```python
from build123d import *

# Parameters (mm, degrees)
LINEAR_AUSTRAGEN1_DEPTH         = 5
M5X0_8_GEWINDEKERNLOCH1_D       = 4.2
M5X0_8_GEWINDEKERNLOCH1_DEPTH   = 14
M5X0_8_GEWINDEKERNLOCH1_TIP     = 1.2618073
SKIZZE5_R                       = 2.5
SCHNITT_LINEAR_AUSTRAGEN1_DEPTH = 825.102693843
LINEARES_MUSTER1_COUNT          = 2
LINEARES_MUSTER1_PITCH          = 60
LINEARES_MUSTER1_COUNT_DIR2     = 2
LINEARES_MUSTER1_PITCH_DIR2     = 75


with BuildPart() as part:
    # Skizze1 → Linear austragen1 (new body)
    with BuildSketch(Plane.XY):
        Polygon((-370.5, 400), (370.5, 400), (370.5, 348), (422.5, 348), (422.5, 360), (708.5, 360), (708.5, 348), (720.5, 348), (720.5, -348), (708.5, -348), (708.5, -360), (422.5, -360), (422.5, -348), (370.5, -348), (370.5, -400), (-370.5, -400), align=None)
    extrude(amount=LINEAR_AUSTRAGEN1_DEPTH)

    # M5x0.8 Gewindekernloch1
    with Locations(Plane(origin=(345.5, 206, 5), x_dir=(1, 0, 0), z_dir=(0, 0, 1))):
        with Locations((0, 0), (-100, 0), (-100, -100), (0, -100), (0, -312), (-100, -312), (0, -412), (-100, -412)):
            Hole(M5X0_8_GEWINDEKERNLOCH1_D / 2, depth=M5X0_8_GEWINDEKERNLOCH1_DEPTH)
            with Locations((0, 0, -(M5X0_8_GEWINDEKERNLOCH1_DEPTH + M5X0_8_GEWINDEKERNLOCH1_TIP / 2))):  # 118° drill point
                Cone(0, M5X0_8_GEWINDEKERNLOCH1_D / 2, M5X0_8_GEWINDEKERNLOCH1_TIP, mode=Mode.SUBTRACT)

    # Skizze5 → Schnitt-Linear austragen1 (cut, through all)
    with BuildSketch(Plane.XY.offset(5)):
        with Locations((240.5, 183)):
            Circle(SKIZZE5_R)
        with Locations((240.5, 129.152)):
            Circle(SKIZZE5_R)
        with Locations((240.5, -128.952)):
            Circle(SKIZZE5_R)
        with Locations((240.5, -182.8)):
            Circle(SKIZZE5_R)
    extrude(amount=-SCHNITT_LINEAR_AUSTRAGEN1_DEPTH, mode=Mode.SUBTRACT)

    # Skizze8 → Ø6.5 (6.5) Durchmesser Bohrung1 (revolve, cut)
    with BuildSketch(Plane(origin=(427.5, 186, 5), x_dir=(0, -1, 0), z_dir=(1, 0, 0))):
        Polygon((0, 0), (0, 21.952797012), (3.25, 20), (3.25, 0), align=None)
    f_6_5_6_5_durchmesser_bohrung1 = revolve(axis=Axis((427.5, 186, 11.35), (0, 0, -1)), mode=Mode.SUBTRACT)

    # Lineares Muster1: 6.5 _6.5_ Durchmesser Bohrung1 2 × 2
    with Locations(*[(j * LINEARES_MUSTER1_PITCH_DIR2, -i * LINEARES_MUSTER1_PITCH, 0) for i in range(LINEARES_MUSTER1_COUNT) for j in range(LINEARES_MUSTER1_COUNT_DIR2) if (i, j) != (0, 0)]):
        add(f_6_5_6_5_durchmesser_bohrung1, mode=Mode.SUBTRACT)

    # Spiegeln1: Ø6.5 (6.5) Durchmesser Bohrung1 across plane
    add(f_6_5_6_5_durchmesser_bohrung1.mirror(Plane.ZX), mode=Mode.SUBTRACT)

    # Spiegeln1 copy 1 sketch → Spiegeln1 copy 1 (revolve, cut)
    with BuildSketch(Plane(origin=(502.5, -186, 5), x_dir=(0, 1, 0), z_dir=(1, 0, 0))):
        Polygon((0, 0), (0, -21.952797012), (3.25, -20), (3.25, 0), align=None)
    revolve(axis=Axis((502.5, -186, 11.35), (0, 0, 1)), mode=Mode.SUBTRACT)

    # Spiegeln1 copy 2 sketch → Spiegeln1 copy 2 (revolve, cut)
    with BuildSketch(Plane(origin=(427.5, -126, 5), x_dir=(0, 1, 0), z_dir=(1, 0, 0))):
        Polygon((0, 0), (0, -21.952797012), (3.25, -20), (3.25, 0), align=None)
    revolve(axis=Axis((427.5, -126, 11.35), (0, 0, 1)), mode=Mode.SUBTRACT)

    # Spiegeln1 copy 3 sketch → Spiegeln1 copy 3 (revolve, cut)
    with BuildSketch(Plane(origin=(502.5, -126, 5), x_dir=(0, 1, 0), z_dir=(1, 0, 0))):
        Polygon((0, 0), (0, -21.952797012), (3.25, -20), (3.25, 0), align=None)
    revolve(axis=Axis((502.5, -126, 11.35), (0, 0, 1)), mode=Mode.SUBTRACT)


solid = part.part
```
Check sheet for the modelled part. Datum: model origin and axes. Units: mm. Coordinates: 2 decimals unless noted, no trailing zeros. Write each loop counter-clockwise with the first axis right and the second up, starting at its lowest first coordinate (ties: lowest second). Pieces come first, ordered by that corner, then holes. Notation, with made-up numbers: M 79,68.5 L 113,68.5 A23 ccw 113,97.5 Z; hole C 13.5,70.5 d2. An arc over 180 degrees is marked long. Write item = value, one per line. Start each with the question number.
1. Sectioned sample at A-A (x = 472.5). Record the cut outline in (y, z).
2. Go/stop test with a flat-tipped pin: pin 1 (1 mm diameter, centred on x = 535, z = 1, fed in from -Y). Record where the tip stops, or that it passes through.
3. Sectioned sample at B-B (z = 3.9). State how many separate pieces and enclosed holes the cut face has, then the cut area to 3 significant figures.
4. Thickness scan on probe 1 along Y at (x, z) = (345.5, 1.65); probe 2 along X at (y, z) = (-206, 2.35); probe 3 along Y at (x, z) = (502.5, 2.2). Record the ranges inside material, lowest first.
The answers:
q1.outline = M -360,0 L 360,0 L 360,5 L -360,5 Z
q2.pin_1 = -360
q3.separate_pieces = 1
q3.enclosed_holes = 20
q3.area = 843,000 mm²
q4.probe_1 = -400 to -208.1, -203.9 to -108.1, -103.9 to 103.9, 108.1 to 203.9, 208.1 to 400
q4.probe_2 = -370.5 to 243.4, 247.6 to 343.4, 347.6 to 720.5
q4.probe_3 = -360 to -189.25, -182.75 to -129.25, -122.75 to 122.75, 129.25 to 182.75, 189.25 to 360
